Work out the finished part from the listing and answer in its coordinate system (mm). Face numbers are marked on the shaded views. A direction names the side the tool comes from. Round coordinates to 2 decimals unless told otherwise and drop trailing zeros. Loops run counter-clockwise (first coordinate to the right, second up) from the corner with the lowest first, then second, coordinate; pieces in that order, holes last. Notation, with made-up numbers: (48, 32.25) - (72, 32.25) arc R3 ccw to (72, 36.25) - close; hole circle Ø8 at (43.25, -11.5). An arc over 180 degrees is marked (long way). Answer as CSV lines item,"result". Start each with the question number.
Q1. Section C-C on z = -3.5 is taken. Write down the section's boundary in (x, y).
Q2. Section A-A on x = 0.1 is taken. Write down the section's boundary in (y, z).
Q3. Straight lines are drawn through the part: L1, parallel to X at y = 3, z = 2; L2, parallel to Z at x = 9, y = -6. For each, find the intervals that lie inside material, in ascending order. Write a range as [from, to].
Q4. For the marked faces 1 and 2, determine the directions among +Z, -Z, +X, -X, +Y, -Y from which every point of the face is accessible in a straight line to the end or side of a thin tool.
Q5. Each of these flat-tipped pins is pushed along its axis until it touches: pin 1 Ø1.2 at (x, z) = (9.5, 8.5) entering from +Y; pin 2 Ø3.5 at (x, y) = (-8.5, 10) entering from -Z. Where does it stop, or does it pass through?
Q6. Section D-D on x = 5.5 is taken. Write down the section's boundary in (y, z), then the cut area to 3 significant figures.
Q7. The mould has two halves that part along X. Classify the marked faces 3, 4, 5 and 6: +X half, -X half, draft (parallel to the pull), parting line (faces both ways), or undercut.
Q8. Section B-B on y = 0.3 is taken. Write down the section's boundary in (x, z).
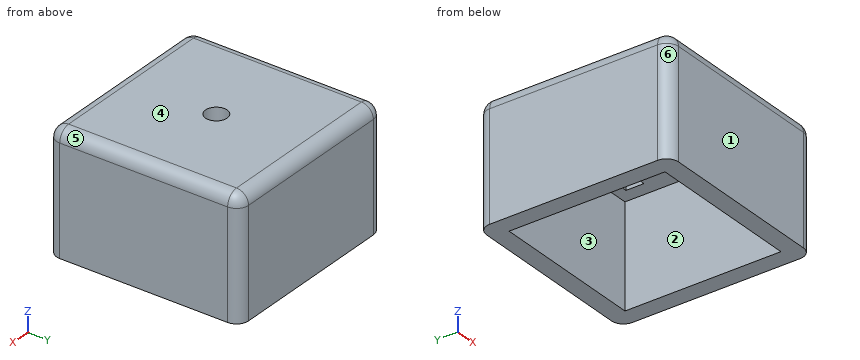
```python
from build123d import *

# Parameters (mm, degrees)
CYLINDER001_R     = 1.8
CYLINDER001_DEPTH = 3
BOX006_W          = 3
BOX006_H          = 3
BOX006_DEPTH      = 3
BOX005_W          = 3
BOX005_H          = 3
BOX005_DEPTH      = 3
BOX003_W          = 3
BOX003_H          = 3
BOX003_DEPTH      = 3
BOX004_W          = 3
BOX004_H          = 3
BOX004_DEPTH      = 3
BOX002_W          = 3
BOX002_H          = 3
BOX002_DEPTH      = 3
BOX_W             = 26
BOX_H             = 26
BOX_DEPTH         = 17
BOX001_W          = 32
BOX001_H          = 32
BOX001_DEPTH      = 20
FILLET003_R       = 2


with BuildPart() as obj1:
    # Cylinder001 → Cylinder001 (new body)
    with BuildSketch(Plane(origin=(0.1, 0.3, 7), x_dir=(1, 0, 0), z_dir=(0, 0, 1))):
        Circle(CYLINDER001_R)
    extrude(amount=CYLINDER001_DEPTH)


with BuildPart() as l5:
    # Box006 → Box006 (new body)
    with BuildSketch(Plane(origin=(7.67, 8.11, 6.5), x_dir=(1, 0, 0), z_dir=(0, 0, 1))):
        with Locations((1.5, 1.5)):
            Rectangle(BOX006_W, BOX006_H)
    extrude(amount=BOX006_DEPTH)


with BuildPart() as l4:
    # Box005 → Box005 (new body)
    with BuildSketch(Plane(origin=(3.1, 8.11, 6.5), x_dir=(1, 0, 0), z_dir=(0, 0, 1))):
        with Locations((1.5, 1.5)):
            Rectangle(BOX005_W, BOX005_H)
    extrude(amount=BOX005_DEPTH)


with BuildPart() as l2:
    # Box003 → Box003 (new body)
    with BuildSketch(Plane(origin=(-6.04, 8.11, 6.5), x_dir=(1, 0, 0), z_dir=(0, 0, 1))):
        with Locations((1.5, 1.5)):
            Rectangle(BOX003_W, BOX003_H)
    extrude(amount=BOX003_DEPTH)


with BuildPart() as l3:
    # Box004 → Box004 (new body)
    with BuildSketch(Plane(origin=(-1.47, 8.11, 6.5), x_dir=(1, 0, 0), z_dir=(0, 0, 1))):
        with Locations((1.5, 1.5)):
            Rectangle(BOX004_W, BOX004_H)
    extrude(amount=BOX004_DEPTH)


with BuildPart() as fusion:
    # Box002 → Box002 (new body)
    with BuildSketch(Plane(origin=(-10.61, 8.11, 6.5), x_dir=(1, 0, 0), z_dir=(0, 0, 1))):
        with Locations((1.5, 1.5)):
            Rectangle(BOX002_W, BOX002_H)
    extrude(amount=BOX002_DEPTH)

    # Fusion: union L5, L4, L2, L3
    add(l5.part)
    add(l4.part)
    add(l2.part)
    add(l3.part)


with BuildPart() as maininside:
    # Box → Box (new body)
    with BuildSketch(Plane(origin=(-13, -13, -10), x_dir=(1, 0, 0), z_dir=(0, 0, 1))):
        with Locations((13, 13)):
            Rectangle(BOX_W, BOX_H)
    extrude(amount=BOX_DEPTH)


with BuildPart() as fillet003:
    # Box001 → Box001 (new body)
    with BuildSketch(Plane(origin=(-16, -16, -10), x_dir=(1, 0, 0), z_dir=(0, 0, 1))):
        with Locations((16, 16)):
            Rectangle(BOX001_W, BOX001_H)
    extrude(amount=BOX001_DEPTH)

    # Cut: cut MainInside
    add(maininside.part, mode=Mode.SUBTRACT)

    # Cut001: cut Fusion
    add(fusion.part, mode=Mode.SUBTRACT)

    # Cut002: cut obj1
    add(obj1.part, mode=Mode.SUBTRACT)

    # Fillet003
    fillet003_edges = [fillet003.edges().sort_by_distance(p)[0] for p in [
        (-16, -16, 0),
        (-16, 0, 10),
        (-16, 16, 0),
        (16, -16, 0),
        (0, -16, 10),
        (0, 16, 10),
        (16, 0, 10),
        (16, 16, 0),
    ]]
    fillet(fillet003_edges, radius=FILLET003_R)


solid = fillet003.part
```
Findings:
1,outline,"(-16, -14) arc R2 ccw to (-14, -16) - (14, -16) arc R2 ccw to (16, -14) - (16, 14) arc R2 ccw to (14, 16) - (-14, 16) arc R2 ccw to (-16, 14) - close; hole (-13, -13) - (13, -13) - (13, 13) - (-13, 13) - close"
2,outline,"(-16, -10) - (-13, -10) - (-13, 7) - (-1.5, 7) - (-1.5, 10) - (-14, 10) arc R2 ccw to (-16, 8) - close; (2.1, 7) - (8.11, 7) - (8.11, 9.5) - (11.11, 9.5) - (11.11, 7) - (13, 7) - (13, -10) - (16, -10) - (16, 8) arc R2 ccw to (14, 10) - (2.1, 10) - close"
3,L1,"x = [-16, -13], [13, 16]"
3,L2,"z = [7, 10]"
4,face 1,"+Z, -Z, +X, -X, -Y"
4,face 2,"-Z"
5,pin 1,"stops at y = 16"
5,pin 2,"stops at z = 7"
6,outline,"(-16, -10) - (-13, -10) - (-13, 7) - (8.11, 7) - (8.11, 9.5) - (11.11, 9.5) - (11.11, 7) - (13, 7) - (13, -10) - (16, -10) - (16, 8) arc R2 ccw to (14, 10) - (-14, 10) arc R2 ccw to (-16, 8) - close"
6,area,"189 mm^2"
7,face 3,"undercut"
7,face 4,"draft"
7,face 5,"+X half"
7,face 6,"-X half"
8,outline,"(-16, -10) - (-13, -10) - (-13, 7) - (-1.7, 7) - (-1.7, 10) - (-14, 10) arc R2 ccw to (-16, 8) - close; (1.9, 7) - (13, 7) - (13, -10) - (16, -10) - (16, 8) arc R2 ccw to (14, 10) - (1.9, 10) - close"
